Verification items for the finished model (mm, model axes). A direction names the side the tool comes from. Round coordinates to 2 decimals unless told otherwise and drop trailing zeros. Write each loop counter-clockwise with the first axis right and the second up, starting at its lowest first coordinate (ties: lowest second). Pieces come first, ordered by that corner, then holes. Notation, with made-up numbers: (23.5, 41.5) - (63.5, 41.5) arc R23 cw to (63.5, 79.5) - close; hole circle Ø7 at (83, 65.5). An arc over 180 degrees is marked (long way). Answer as a JSON object with one key per item and string values.
Autodesk Inventor part; units mm, degrees
ref_plane "YZ Plane" through (0, 0, 0) normal (1, 0, 0) x (0, 1, 0)
ref_plane "XZ Plane" through (0, 0, 0) normal (0, 1, 0) x (-1, 0, 0)
ref_plane "XY Plane" through (0, 0, 0) normal (0, 0, 1) x (1, 0, 0)
sketch "Sketch1" plane through (0, 0, 0) normal (0, 1, 0) x (-1, 0, 0)
  line L0 (0, 0) -> (50, 0)
  line L1 (50, 0) -> (50, 3)
  line L2 (0, 0) -> (0, 50)
  line L3 (0, 50) -> (3, 50)
  line L4 (3, 50) -> (3, 3)
  line L5 (3, 3) -> (50, 3)
  dimension "d0" = 50
  dimension "d1" = 3
  dimension "d2" = 50
  dimension "d3" = 3
extrude "Extrusion1" add sketch "Sketch1" along normal blind 660.4
sketch "Sketch5" plane through (-3, 0, 3) normal (-1, 0, 0) x (0, 0, 1)
  circle A0 centre (24.5, 59.2629) radius 4.8387
  circle A1 centre (24.5, 149.2629) radius 4.8387
  circle A2 centre (24.5, 219.0371) radius 4.8387
  circle A3 centre (24.5, 309.0371) radius 4.8387
  line L0 (0, 0) -> (47, 0)
  line L1 (0, 0) -> (0, 660.4)
  line L2 (-136.6387, 184.15) -> (192.6114, 184.15) construction
  line L3 (47, 0) -> (47, 660.4)
  line L4 (-3, 0) -> (-3, 660.4) construction
  dimension "d68" = 90
  dimension "d70" = 90
  dimension "d71" = 69.7742
  dimension "d72" = 184.15
  dimension "d73" = 34.8871
  dimension "d74" = 34.8871
  dimension "d78" = 59.2629
  dimension "d79" = 50
  dimension "d102" = 22.5
sketch "Sketch6" plane through (-50, 0, 3) normal (0, 0, 1) x (1, 0, 0)
  line L0 (0, 0) -> (47, 0)
  line L1 (47, 0) -> (47, 660.4)
  line L2 (0, 660.4) -> (47, 660.4)
  line L3 (0, 0) -> (0, 660.4)
  line L4 (0, 0) -> (47, 0)
  line L5 (47, 0) -> (47, 660.4)
  line L6 (0, 660.4) -> (47, 660.4)
  line L7 (0, 0) -> (0, 660.4)
  line L8 (50, 0) -> (50, 660.4)
  line L9 (47, 660.4) -> (50, 660.4)
  line L10 (0, 644.4) -> (50, 644.4) construction
  circle A0 centre (6.35, 644.4) radius 3.175
  circle A1 centre (40.65, 644.4) radius 3.175
  line L11 (50, 16) -> (0, 16) construction
  circle A2 centre (40.65, 16) radius 3.175
  circle A3 centre (6.35, 16) radius 3.175
  dimension "d80" = 16
  dimension "d81" = 6.35
  dimension "d82" = 6.35
  dimension "d83" = 6.35
  dimension "d84" = 6.35
  dimension "d85" = 16
  dimension "d86" = 6.35
  dimension "d87" = 6.35
hole "Hole1" at (-9.35, 644.4, 3) at (-43.65, 644.4, 3) at (-9.35, 16, 3) at (-43.65, 16, 3) direction (0, 0, -1) diameter 6.35 depth 3 tip angle 118
hole "Hole2" at (-3, 59.2629, 27.5) at (-3, 149.2629, 27.5) at (-3, 219.0371, 27.5) at (-3, 309.0371, 27.5) direction (1, 0, 0) diameter 12 depth 3 tip angle 118
equation "\"d68\" = d70"
equation "\"d73\" = 0.5 * d71"
equation "\"d74\" = 0.5 * d71"
properties part number "26in Angle Channel CIM Mount Left" material "Aluminum 6061"
1. Mould release check, pull along Y, two halves, no side actions. Record for faces 1 (the face through (-1.48, 303.09, 26.72)), 2 (the face through (-26, 326, 3)), 3 (the face through (-2.7, 0, 14)): released by +Y, released by -Y, zero draft, split by the parting line, or undercut.
Completed:
{"face 1": "undercut", "face 2": "zero draft", "face 3": "released by -Y"}
2. Access from +Z, -Z, +X, -X, +Y, -Y to the whole of each face (thin tool, end or side, straight path). Record for faces 4 (the face through (-3, 326, 27)), 5 (the face through (-1.48, 155.12, 26.2)).
Completed:
{"face 4": "+Z, -X, +Y, -Y", "face 5": "+X, -X"}
3. Cross-section at C-C (x = -24). Record the boundary of the cut face in (y, z), plus the area to 3 significant figures.
Completed:
{"outline": "(0, 0) - (660.4, 0) - (660.4, 3) - (0, 3) - close", "area": "1,980 mm^2"}
4. Go/stop test with flat-tipped pins: pin 1 (14 mm diameter, centred on x = -20, y = 227.5, fed in from +Z); pin 2 (23.5 mm diameter, centred on y = 228, z = 25.5, fed in from -X); pin 3 (7.5 mm diameter, centred on x = -9.35, y = 16, fed in from -Z); pin 4 (4 mm diameter, centred on x = -43.65, y = 644.4, fed in from -Z). Record where each tip stops, or that it passes through.
Completed:
{"pin 1": "stops at z = 3", "pin 2": "stops at x = -3", "pin 3": "stops at z = 0", "pin 4": "passes through"}
5. Cross-section at B-B (y = 525). Record the boundary of the cut face in (x, z), plus the area to 3 significant figures.
Completed:
{"outline": "(-50, 0) - (0, 0) - (0, 50) - (-3, 50) - (-3, 3) - (-50, 3) - close", "area": "291 mm^2"}
6. Cross-section at A-A (z = 27.5). Record the boundary of the cut face in (x, y), plus the area to 3 significant figures.
Completed:
{"outline": "(-3, 0) - (0, 0) - (0, 53.26) - (-3, 53.26) - close; (-3, 65.26) - (0, 65.26) - (0, 143.26) - (-3, 143.26) - close; (-3, 155.26) - (0, 155.26) - (0, 213.04) - (-3, 213.04) - close; (-3, 225.04) - (0, 225.04) - (0, 303.04) - (-3, 303.04) - close; (-3, 315.04) - (0, 315.04) - (0, 660.4) - (-3, 660.4) - close", "area": "1,840 mm^2"}
7. Material ranges on probe 1 along Y at (x, z) = (-2, 27); probe 2 along Y at (x, z) = (-43.65, 1.85) (3 decimals); probe 3 along Y at (x, z) = (-1.6, 27.5), recorded low to high. Write a range as from..to.
Completed:
{"probe 1": "y = 0..53.28, 65.24..143.28, 155.24..213.06, 225.02..303.06, 315.02..660.4", "probe 2": "y = 0..12.825, 19.175..641.225, 647.575..660.4", "probe 3": "y = 0..53.26, 65.26..143.26, 155.26..213.04, 225.04..303.04, 315.04..660.4"}
